Check sheet for the modelled part. Datum: model origin and axes. Units: mm. A direction names the side the tool comes from. Round coordinates to 2 decimals unless told otherwise and drop trailing zeros. Write each loop counter-clockwise with the first axis right and the second up, starting at its lowest first coordinate (ties: lowest second). Pieces come first, ordered by that corner, then holes. Notation, with made-up numbers: M -22,84.25 L 2,84.25 A18 ccw 2,105.25 Z; hole C 54,16 d7. An arc over 180 degrees is marked long. Answer in a Markdown table with one row per item.
Autodesk Inventor part; units mm, degrees
ref_plane "YZ Plane" through (0, 0, 0) normal (1, 0, 0) x (0, 1, 0)
ref_plane "XZ Plane" through (0, 0, 0) normal (0, 1, 0) x (-1, 0, 0)
ref_plane "XY Plane" through (0, 0, 0) normal (0, 0, 1) x (1, 0, 0)
sketch "Skizze1" plane through (0, 0, 0) normal (0, 0, 1) x (1, 0, 0)
  line L0 (0, 0) -> (135, 0)
  line L1 (135, 0) -> (135, -60)
  line L2 (135, -60) -> (0, -60)
  line L3 (0, -60) -> (0, 0)
  dimension "d0" = 135
  dimension "d1" = 60
extrude "Extrusion1" add sketch "Skizze1" along normal blind 40
chamfer "Fase1" distance 38 angle 30 1 edges at (0, -30, 40) measured on face at (0, -20, 13.3333)
shell "Wandung1" thickness 2.5 removed faces 1 at (59.626207, -20, 40)
sketch "Skizze2" plane through (0, 0, 40) normal (0, 0, 1) x (1, 0, 0)
  line L0 (24.826062, -57.5) -> (24.826062, -2.5)
  line L1 (24.826062, -2.5) -> (24.826062, 0)
  line L2 (24.826062, 0) -> (24.826062, -57.5)
  line L3 (24.826062, -57.5) -> (24.826062, -60)
  line L4 (32.285534, -57.5) -> (32.285534, -2.5)
  line L5 (32.285534, -2.5) -> (132.5, -2.5)
  line L6 (132.5, -2.5) -> (132.5, -57.5)
  line L7 (132.5, -57.5) -> (32.285534, -57.5)
  line L8 (21.290528, -60) -> (21.290528, 0)
  line L9 (21.290528, -60) -> (24.826062, -60)
  line L10 (135.042932, -60) -> (135.042932, 0)
  line L11 (135.042932, 0) -> (24.826062, 0)
  line L12 (24.826062, -60) -> (135.042932, -60)
  line L13 (24.826062, 0) -> (21.290528, 0)
  point P0 (0, 0)
  point P1 (32.285534, -2.5)
extrude "Extrusion2" cut sketch "Skizze2" against normal blind 9.5 contours L0 L1 L11 L10 L12 L3
sketch "Skizze3" plane through (0, -60, 0) normal (0, -1, 0) x (1, 0, 0)
  point P0 (0, 0)
  point P1 (100.666226, 14.858037)
hole "Bohrung1" at (100.666226, -60, 14.858037) direction (0, 1, 0) diameter 2 depth 8 tip angle 118
sketch "Skizze4" plane through (132.5, -57.5, 2.5) normal (-1, 0, 0) x (0, 0, 1)
  line L0 (22.221117, 33.89428) -> (25.5, 33.89428)
  line L1 (25.5, 33.89428) -> (25.5, 21.10572)
  line L2 (25.5, 21.10572) -> (22.221117, 21.10572)
  line L3 (22.221117, 21.10572) -> (22.221117, 33.89428)
  line L4 (0, 0) -> (0, 55)
  line L5 (0, 27.5) -> (28, 27.5)
  line L6 (28, 0) -> (28, 55)
  line L7 (28, 57.5) -> (28, -2.5)
  point P0 (-2.5, 57.5)
  dimension "d22" = 2.5
extrude "Extrusion3" cut sketch "Skizze4" against normal blind 1
sketch "Skizze5" plane through (0, -60, 0) normal (0, -1, 0) x (1, 0, 0)
  line L0 (132.5, 30.5) -> (24.826062, 30.5)
  line L1 (32.285534, 30.5) -> (19.341234, 30.5)
  line L2 (19.341234, 30.5) -> (24.826062, 40)
  line L3 (3.175426, 2.5) -> (24.826062, 40)
  line L4 (24.826062, 40) -> (32.013518, 40)
  line L5 (32.013518, 40) -> (32.013518, 30.5)
  point P0 (0, 0)
  point P1 (2.5, 4.827159)
  point P2 (23.251035, 30.965501)
  point P3 (127.540528, 30.5)
  point P4 (24.826062, 40)
extrude "Extrusion4" cut sketch "Skizze5" against normal through all
sketch "Skizze6" plane through (0, -60, 0) normal (0, -1, 0) x (1, 0, 0)
  circle A0 centre (100.666226, 14.858037) radius 1
  line L0 (124.166226, 9.858037) -> (123.166226, 9.858037)
  line L1 (123.166226, 9.858037) -> (123.166226, 19.858037)
  line L2 (123.166226, 19.858037) -> (124.166226, 19.858037)
  line L3 (124.166226, 19.858037) -> (124.166226, 9.858037)
  line L4 (100.666226, 14.858037) -> (116.026843, 14.858037)
  point P0 (0, 0)
  dimension "d23" = 1
  dimension "d24" = 10
  dimension "d25" = 22.5
extrude "Extrusion5" cut sketch "Skizze6" against normal up to surface (2.5 mm away) contours L0 L1 L2 L3
sketch "Skizze7" plane through (0, 0, 0) normal (0, 0, -1) x (-1, 0, 0)
  line L0 (0, -36) -> (6.514704, -36)
  line L1 (12.514704, -30) -> (12.514704, -30)
  line L2 (6.514704, -24) -> (0, -24)
  line L3 (0, -24) -> (0, -36)
  line L4 (-21.93931, -60) -> (-21.93931, 0)
  line L5 (-21.93931, -30) -> (18.562445, -30)
  circle A0 centre (6.514704, -30) radius 3
  arc A1 (6.514704, -36) -> (12.514704, -30) centre (6.514704, -30) ccw
  arc A2 (12.514704, -30) -> (6.514704, -24) centre (6.514704, -30) ccw
  point P0 (0, 0)
  point P1 (12.514704, -30)
  dimension "d28" = 6
  dimension "d29" = 6
  dimension "d30" = 6
  dimension "d31" = 6
extrude "Extrusion6" add sketch "Skizze7" against normal blind 2 contours L3 L5 A0 A1 L0 | L3 L2 A2 L5 A0
fillet "Rundung1" radius 4.75 2 edges at (0, -24, 1) (0, -36, 1)
fillet "Rundung2" radius 4.75 7 edges at (21.9393, -30, 40) (10.9697, -60, 21) (10.9697, 0, 21) (135, 0, 15.25) (135, -60, 15.25) (132.5, -57.5, 16.5) (132.5, -2.5, 16.5)
properties part number "Case"
1. Section check B-B, the plane x = 62.5. Record the cut outline in (y, z), and give its area (3 significant figures).
Found:
| item | result |
|---|---|
| outline | M -60,0 L 0,0 L 0,30.5 L -2.5,30.5 L -2.5,2.5 L -57.5,2.5 L -57.5,30.5 L -60,30.5 Z |
| area | 290 mm2 |
2. Draft check along Z on faces 5 (the face through (60, -30, 0)), 6 (the face through (132.5, -30, 16)), 7 (the face through (10.428, -29.647, 20.062)), 8 (the face through (133.5, -30, 26)). Enter one of: +Z half, -Z half, draft (parallel to the pull), parting line (faces both ways), or undercut.
Found:
| item | result |
|---|---|
| face 5 | -Z half |
| face 6 | draft |
| face 7 | +Z half |
| face 8 | undercut |
3. Access from +Z, -Z, +X, -X, +Y, -Y to the whole of each face (thin tool, end or side, straight path). Record for faces 1 (the face through (-4, -27, 2)), 2 (the face through (67, -30, 2.5)), 3 (the face through (131.072, -56.145, 16.696)), 4 (the face through (123.166, -59, 15)).
Found:
| item | result |
|---|---|
| face 1 | +Z, -X, +Y, -Y |
| face 2 | none |
| face 3 | +Z |
| face 4 | -Y |
4. Scan lines: L1, parallel to X at y = -30, z = 1.55; L2, parallel to Y at x = 55, z = 28.5; L3, parallel to Z at x = 81.5, y = -6. Record each from-to range of solid material in increasing order.
Found:
| item | result |
|---|---|
| L1 | x = -12.51 to -9.51, -3.51 to 135 |
| L2 | y = -60 to -57.5, -2.5 to 0 |
| L3 | z = 0 to 2.5 |
5. Go/stop test with flat-tipped pins: pin 1 (1.4 mm diameter, centred on x = -5.5, z = 1, fed in from +Y); pin 2 (0.8 mm diameter, centred on x = 133, z = 26, fed in from +Y); pin 3 (3.5 mm diameter, centred on y = -29.5, z = 27, fed in from -X). Record where each tip stops, or that it passes through.
Found:
| item | result |
|---|---|
| pin 1 | stops at y = -24 |
| pin 2 | stops at y = -0.62 |
| pin 3 | stops at x = 13.42 |
6. Section check A-A, the plane y = -30. Record the cut outline in (x, z) (3 decimals).
Found:
| item | result |
|---|---|
| outline | M -12.515,0 L -9.515,0 L -9.515,2 L -12.515,2 Z; M -3.515,0 L 135,0 L 135,30.5 L 132.5,30.5 L 132.5,28 L 133.5,28 L 133.5,24.721 L 132.5,24.721 L 132.5,2.5 L 3.175,2.5 L 24.826,40 L 24.682,40 A4.75 ccw 20.568,37.625 L 0,2 L -3.515,2 Z |
